```python
from build123d import *

# Parameters (mm, degrees)
F0_W      = 101.443342
F0_H      = 12.895348
F1_DEPTH  = 4.064
F2_W      = 12.895348
F2_H      = 4.064
F3_DEPTH  = 4.064
F4_W      = 12.895348
F4_H      = 4.064
F5_DEPTH  = 4.064
F6_W      = 12.9032
F6_H      = 44.474205
F7_DEPTH  = 4.064
F8_W      = 12.9032
F8_H      = 4.064
F9_DEPTH  = 4.064
F10_R     = 3.476261
F11_DEPTH = 6.0198
F12_R     = 1.22642
F13_R     = 1.900656
F14_DEPTH = 0.2794


with BuildPart() as f1:
    # F0 (on Top) → F1 (new body)
    with BuildSketch(Plane.XY):
        Rectangle(F0_W, F0_H)
    extrude(amount=F1_DEPTH)

    # F2 (on face) → F3 (join)
    with BuildSketch(Plane.YZ.offset(50.721671)):
        Polygon((-6.447674, 55.437263), (-6.447674, 4.064), (6.447674, 4.064), (6.447674, 55.437263), (2.940099, 59.015486), (-2.682819, 59.015486), align=None)
        with Locations((0, 2.032)):
            Rectangle(F2_W, F2_H)
    extrude(amount=-F3_DEPTH)

    # F4 (on face) → F5 (join)
    with BuildSketch(Plane(origin=(-50.721671, 0, 0), x_dir=(0, -1, 0), z_dir=(-1, 0, 0))):
        Polygon((-6.734233, 55.44746), (-6.447674, 0), (-6.447674, 4.064), (6.447674, 4.064), (6.447674, 55.44746), (2.663421, 58.72121), (-2.949979, 58.72121), align=None)
        with Locations((0, 2.032)):
            Rectangle(F4_W, F4_H)
    extrude(amount=-F5_DEPTH)

    # F6 (on Top) → F7 (join)
    with BuildSketch(Plane.XY):
        with Locations((0, -28.486697)):
            Rectangle(F6_W, F6_H)
    extrude(amount=F7_DEPTH)

    # F8 (on face) → F9 (join)
    with BuildSketch(Plane.XZ.offset(50.7238)):
        Polygon((-6.4516, 55.4482), (-6.4516, 4.064), (6.4516, 4.064), (6.4516, 55.4482), (2.8067, 58.876424), (-2.8067, 58.876424), align=None)
        with Locations((0, 2.032)):
            Rectangle(F8_W, F8_H)
    extrude(amount=-F9_DEPTH)

    # F10 (on face) → F11 (join)
    with BuildSketch(Plane.XY.offset(4.064)):
        Circle(F10_R)
    extrude(amount=F11_DEPTH)

    # F12
    f12_edges = [f1.edges().sort_by_distance(p)[0] for p in [
        (-46.657671, 0, 4.064),
        (46.657671, 0, 4.064),
        (50.721671, 0, 0),
        (-50.721671, 0, 0),
        (0, -50.7238, 0),
        (0, -46.6598, 4.064),
    ]]
    fillet(f12_edges, radius=F12_R)

    # F13 (on face) → F14 (join)
    with BuildSketch(Plane.XY.offset(10.0838)):
        Circle(F13_R)
    extrude(amount=F14_DEPTH)


solid = f1.part
```
Read the model definition and answer for the solid it produces. Units are mm, in the model's axes. A direction names the side the tool comes from. Round coordinates to 2 decimals unless told otherwise and drop trailing zeros. Write each loop counter-clockwise with the first axis right and the second up, starting at its lowest first coordinate (ties: lowest second). Pieces come first, ordered by that corner, then holes. Notation, with made-up numbers: (32, -24.5) -> (40, -24.5) arc R28 ccw to (40, -5.5) -> close; hole circle Ø7 at (24, 13.25). An arc over 180 degrees is marked (long way). Answer in a Markdown table with one row per item. Add a question column.
1) Determine the mould class of faces 1 (the face through (48.72, 4.72, 57.2)), 2 (the face through (0, 0, 10.363)), 3 (the face through (-4.6, -48.72, 57.19)) for opening direction X: pulls with the +X half, pulls with the -X half, needs draft (parallel to the pull), parting line crosses it, or undercut.
2) Given P1, Ø22, axis at y = -38, z = 28.5, coming from the +X side; P2, Ø4.5, axis at x = -48.5, y = 0.5, coming from the +Z side; P3, Ø14, axis at x = 1.5, z = 21, coming from the +Y side, each flat-ended and moving along its own axis, determine where each tip first touches the part or whether it passes through.
3) Find section C-C, the plane y = 0. Determine the outline of the cut face in (x, z).
4) Find section B-B, the plane z = 21.5. Determine the outline of the cut face in (x, y), and give its area (3 significant figures).
5) Which of the six approach directions +Z, -Z, +X, -X, +Y, -Y give full straight-line access (tool end or side, diameter ignored) to faces 4 (the face through (47, -6.448, 18)), 5 (the face through (-46.658, 0, 36)), 6 (the face through (17, 6.448, 3))?
6) Consider line 1 (X direction, y = -1, z = 35); line 2 (Z direction, x = -1, y = -45); line 3 (Y direction, x = -1, z = 22). Determine where each line is inside the solid, lowest interval first.
7) Find section D-D, the plane z = 34. Determine the outline of the cut face in (x, y), and give its area (3 significant figures).
8) Find section A-A, the plane x = 0. Determine the outline of the cut face in (y, z), and give its area (3 significant figures).
Findings below:
| question | item | result |
|---|---|---|
| 1 | face 1 | needs draft |
| 1 | face 2 | undercut |
| 1 | face 3 | pulls with the -X half |
| 2 | P1 | x = 6.45 |
| 2 | P2 | z = 58.72 |
| 2 | P3 | y = -46.66 |
| 3 | outline | (-50.72, 1.23) arc R1.23 ccw to (-49.5, 0) -> (49.5, 0) arc R1.23 ccw to (50.72, 1.23) -> (50.72, 59.02) -> (46.66, 59.02) -> (46.66, 5.29) arc R1.23 cw to (45.43, 4.06) -> (3.48, 4.06) -> (3.48, 10.08) -> (1.9, 10.08) -> (1.9, 10.36) -> (-1.9, 10.36) -> (-1.9, 10.08) -> (-3.48, 10.08) -> (-3.48, 4.06) -> (-45.43, 4.06) arc R1.23 cw to (-46.66, 5.29) -> (-46.66, 58.72) -> (-50.72, 58.72) -> close |
| 4 | outline | (-50.72, -6.45) -> (-46.66, -6.45) -> (-46.66, 6.56) -> (-50.72, 6.56) -> close; (-6.45, -50.72) -> (6.45, -50.72) -> (6.45, -46.66) -> (-6.45, -46.66) -> close; (46.66, -6.45) -> (50.72, -6.45) -> (50.72, 6.45) -> (46.66, 6.45) -> close |
| 4 | area | 158 mm² |
| 5 | face 4 | +Z, -Z, +X, -Y |
| 5 | face 5 | +Z, +Y, -Y |
| 5 | face 6 | +Z, -Z, +X, +Y |
| 6 | line 1 | -50.72 to -46.66, 46.66 to 50.72 |
| 6 | line 2 | 0 to 4.06 |
| 6 | line 3 | -50.72 to -46.66 |
| 7 | outline | (-50.72, -6.45) -> (-46.66, -6.45) -> (-46.66, 6.62) -> (-50.72, 6.62) -> close; (-6.45, -50.72) -> (6.45, -50.72) -> (6.45, -46.66) -> (-6.45, -46.66) -> close; (46.66, -6.45) -> (50.72, -6.45) -> (50.72, 6.45) -> (46.66, 6.45) -> close |
| 7 | area | 158 mm² |
| 8 | outline | (-50.72, 1.23) arc R1.23 ccw to (-49.5, 0) -> (6.45, 0) -> (6.45, 4.06) -> (3.48, 4.06) -> (3.48, 10.08) -> (1.9, 10.08) -> (1.9, 10.36) -> (-1.9, 10.36) -> (-1.9, 10.08) -> (-3.48, 10.08) -> (-3.48, 4.06) -> (-45.43, 4.06) arc R1.23 cw to (-46.66, 5.29) -> (-46.66, 58.88) -> (-50.72, 58.88) -> close |
| 8 | area | 498 mm² |
